from build123d import *

# Parameters (mm, degrees)
F0_W     = 6
F0_H     = 21.24
F1_DEPTH = 1.5
F2_W     = 6
F2_H     = 6
F3_DEPTH = 5
F4_R     = 1.5
F5_DEPTH = 6


with BuildPart() as f1:
    # F0 (on Top) → F1 (new body)
    with BuildSketch(Plane.XY):
        Rectangle(F0_W, F0_H)
    extrude(amount=F1_DEPTH)

    # F2 (on face) → F3 (join)
    with BuildSketch(Plane.XY.offset(1.5)):
        with Locations((0, 7.62)):
            Rectangle(F2_W, F2_H)
        Rectangle(F2_W, F2_H)
        with Locations((0, -7.62)):
            Rectangle(F2_W, F2_H)
    extrude(amount=F3_DEPTH)

    # F4 (on face) → F5 (join)
    with BuildSketch(Plane.XY.offset(6.5)):
        Circle(F4_R)
        with Locations((0, 7.62)):
            Circle(F4_R)
        with Locations((0, -7.62)):
            Circle(F4_R)
    extrude(amount=F5_DEPTH)


solid = f1.part
Verification items for the finished model (mm, model axes). A direction names the side the tool comes from. Coordinates: 2 decimals unless noted, no trailing zeros. Order: outer loops, then holes, each group sorted by start corner. A loop starts at its lowest first (then second) coordinate and runs counter-clockwise, first axis right, second up. Notation, with made-up numbers: (86, 87) -> (138, 87) arc R24 ccw to (138, 105) -> close; hole circle Ø6 at (-5.5, -35.75). An arc over 180 degrees is marked (long way). Use CSV: the item, a comma, the result in double quotes. Start each with the question number.
Q1. Tool access check on faces 5 (the flat face through (0, 8, 12.5)), 6 (the flat face through (-1, -6, 6.5)), 7 (the flat face through (0, 3, 4)). Record the directions out of +Z, -Z, +X, -X, +Y, -Y that give a thin tool (end or side, any length) a straight path to the whole face; none if there is none.
Q2. Thickness scan on line 1 along Y through (x, z) = (-0.35, 2.75); line 2 along Z through (x, y) = (0.05, -1.75); line 3 along Z through (x, y) = (-2.1, 3.5). Record the ranges inside material, lowest first.
Q3. Depth check by flat-ended pin: P1, Ø2, axis at x = 0.5, z = 9, coming from the +Y side; P2, Ø0.8, axis at x = 1, y = 3.5, coming from the +Z side; P3, Ø1.5, axis at x = 0.5, z = 7.5, coming from the -Y side. Enter the tip coordinate at first touch or a pass-through.
Q4. Section check B-B, the plane z = 2. Record the cut outline in (x, y), and give its area (3 significant figures).
Q5. Section check D-D, the plane x = 2.05. Record the cut outline in (y, z), and give its area (3 significant figures).
Q6. Section check C-C, the plane y = -7.62. Record the cut outline in (x, z).
Q7. Draft check along Y on faces 1 (the flat face through (-3, 0, 3)), 2 (the cylindrical face through (-0.325, -9.084, 9.458)), 3 (the flat face through (0, 4, 1.5)), 4 (the flat face through (0, 10.62, 3)). Enter one of: +Y half, -Y half, draft (parallel to the pull), parting line (faces both ways), or undercut.
Q8. Section check A-A, the plane x = -1.2. Record the cut outline in (y, z), and give its area (3 significant figures).
Returned:
1,face 5,"+Z, +X, -X, +Y, -Y"
1,face 6,"+Z"
1,face 7,"+Z, +X, -X"
2,line 1,"y = -10.62 to -4.62, -3 to 3, 4.62 to 10.62"
2,line 2,"z = 0 to 6.5"
2,line 3,"z = 0 to 1.5"
3,P1,"stops at y = 9.12"
3,P2,"stops at z = 1.5"
3,P3,"stops at y = -9.12"
4,outline,"(-3, -10.62) -> (3, -10.62) -> (3, -4.62) -> (-3, -4.62) -> close; (-3, -3) -> (3, -3) -> (3, 3) -> (-3, 3) -> close; (-3, 4.62) -> (3, 4.62) -> (3, 10.62) -> (-3, 10.62) -> close"
4,area,"108 mm^2"
5,outline,"(-10.62, 0) -> (10.62, 0) -> (10.62, 6.5) -> (4.62, 6.5) -> (4.62, 1.5) -> (3, 1.5) -> (3, 6.5) -> (-3, 6.5) -> (-3, 1.5) -> (-4.62, 1.5) -> (-4.62, 6.5) -> (-10.62, 6.5) -> close"
5,area,"122 mm^2"
6,outline,"(-3, 0) -> (3, 0) -> (3, 6.5) -> (1.5, 6.5) -> (1.5, 12.5) -> (-1.5, 12.5) -> (-1.5, 6.5) -> (-3, 6.5) -> close"
7,face 1,"draft"
7,face 2,"undercut"
7,face 3,"undercut"
7,face 4,"+Y half"
8,outline,"(-10.62, 0) -> (10.62, 0) -> (10.62, 6.5) -> (8.52, 6.5) -> (8.52, 12.5) -> (6.72, 12.5) -> (6.72, 6.5) -> (4.62, 6.5) -> (4.62, 1.5) -> (3, 1.5) -> (3, 6.5) -> (0.9, 6.5) -> (0.9, 12.5) -> (-0.9, 12.5) -> (-0.9, 6.5) -> (-3, 6.5) -> (-3, 1.5) -> (-4.62, 1.5) -> (-4.62, 6.5) -> (-6.72, 6.5) -> (-6.72, 12.5) -> (-8.52, 12.5) -> (-8.52, 6.5) -> (-10.62, 6.5) -> close"
8,area,"154 mm^2"
